Input: part model. Units: mm. Frame: model coordinates. A direction names the side the tool comes from. Round coordinates to 2 decimals unless told otherwise and drop trailing zeros. Loops run counter-clockwise (first coordinate to the right, second up) from the corner with the lowest first, then second, coordinate; pieces in that order, holes last. Notation, with made-up numbers: (23, 51) -> (42, 51) arc R7 cw to (42, 55) -> close; hole circle Ø7 at (39, 34.5). An arc over 180 degrees is marked (long way). Answer as a JSON object with one key per item and string values. Group by question number.
Item 1: Set-up query: faces 5 (the flat face through (155, 18, 3.175)), 6 (the flat face through (88, 0, 3)). Return all of +Z, -Z, +X, -X, +Y, -Y with unobstructed straight access to the full face (end or side cutting, diameter ignored); none if empty.
Item 2: Material intervals for line 1 (Y direction, x = 20, z = 4.65); line 2 (Z direction, x = 114.5, y = 15.25) (3 decimals), sorted ascending. Write a range as [from, to].
Item 3: Draft query along X for faces 1 (the flat face through (0, 13, 3)), 2 (the flat face through (115, 7, 3.175)), 3 (the flat face through (88, 13, 5.715)), 4 (the flat face through (76, 18, 3.175)). Return one class per face: released by +X, released by -X, zero draft, split by the parting line, or undercut.
Item 4: Section query B-B on z = 4.75. Count the separate pieces of the cut face and the enclosed holes in it, and give its area (3 significant figures).
Item 5: Pin query (flat end, axial travel): pin 1 (6 mm diameter, centred on x = 107, y = 6, fed in from -Z); pin 2 (3 mm diameter, centred on x = 62, y = 18, fed in from +Z) (3 decimals). Return the tip coordinate at first contact, or that it passes through.
Item 6: Section query A-A on x = 156. Return loops of the section in (y, z) (3 decimals).
from build123d import *

# Parameters (mm, degrees)
F0_W     = 177.8
F0_H     = 25.4
F1_DEPTH = 3.175
F2_W     = 177.8
F2_H     = 25.4
F2_W_2   = 6.489529
F2_H_2   = 6.479562
F3_DEPTH = 2.54


with BuildPart() as f1:
    # F0 (on Top) → F1 (new body)
    with BuildSketch(Plane.XY):
        with Locations((88.9, 12.7)):
            Rectangle(F0_W, F0_H)
    extrude(amount=F1_DEPTH)

    # F2 (on face) → F3 (join)
    with BuildSketch(Plane.XY.offset(3.175)):
        with Locations((88.9, 12.7)):
            Rectangle(F2_W, F2_H)
        with Locations((9.734293, 7.034986)):
            Rectangle(F2_W_2, F2_H_2, mode=Mode.SUBTRACT)
        with Locations((22.942293, 7.034986)):
            Rectangle(F2_W_2, F2_H_2, mode=Mode.SUBTRACT)
        with Locations((36.150294, 7.034986)):
            Rectangle(F2_W_2, F2_H_2, mode=Mode.SUBTRACT)
        with Locations((49.358294, 7.034986)):
            Rectangle(F2_W_2, F2_H_2, mode=Mode.SUBTRACT)
        with Locations((62.566294, 7.034986)):
            Rectangle(F2_W_2, F2_H_2, mode=Mode.SUBTRACT)
        with Locations((75.774293, 7.034986)):
            Rectangle(F2_W_2, F2_H_2, mode=Mode.SUBTRACT)
        with Locations((88.982293, 7.034986)):
            Rectangle(F2_W_2, F2_H_2, mode=Mode.SUBTRACT)
        with Locations((102.190293, 7.034986)):
            Rectangle(F2_W_2, F2_H_2, mode=Mode.SUBTRACT)
        with Locations((115.398293, 7.034986)):
            Rectangle(F2_W_2, F2_H_2, mode=Mode.SUBTRACT)
        with Locations((128.606293, 7.034986)):
            Rectangle(F2_W_2, F2_H_2, mode=Mode.SUBTRACT)
        with Locations((141.814293, 7.034986)):
            Rectangle(F2_W_2, F2_H_2, mode=Mode.SUBTRACT)
        with Locations((155.022293, 7.034986)):
            Rectangle(F2_W_2, F2_H_2, mode=Mode.SUBTRACT)
        with Locations((168.230293, 7.034986)):
            Rectangle(F2_W_2, F2_H_2, mode=Mode.SUBTRACT)
        with Locations((9.734293, 18.350219)):
            Rectangle(F2_W_2, F2_H_2, mode=Mode.SUBTRACT)
        with Locations((22.942293, 18.350219)):
            Rectangle(F2_W_2, F2_H_2, mode=Mode.SUBTRACT)
        with Locations((36.150294, 18.350219)):
            Rectangle(F2_W_2, F2_H_2, mode=Mode.SUBTRACT)
        with Locations((49.358294, 18.350219)):
            Rectangle(F2_W_2, F2_H_2, mode=Mode.SUBTRACT)
        with Locations((62.566294, 18.350219)):
            Rectangle(F2_W_2, F2_H_2, mode=Mode.SUBTRACT)
        with Locations((75.774293, 18.350219)):
            Rectangle(F2_W_2, F2_H_2, mode=Mode.SUBTRACT)
        with Locations((88.982293, 18.350219)):
            Rectangle(F2_W_2, F2_H_2, mode=Mode.SUBTRACT)
        with Locations((102.190293, 18.350219)):
            Rectangle(F2_W_2, F2_H_2, mode=Mode.SUBTRACT)
        with Locations((115.398293, 18.350219)):
            Rectangle(F2_W_2, F2_H_2, mode=Mode.SUBTRACT)
        with Locations((128.606293, 18.350219)):
            Rectangle(F2_W_2, F2_H_2, mode=Mode.SUBTRACT)
        with Locations((141.814293, 18.350219)):
            Rectangle(F2_W_2, F2_H_2, mode=Mode.SUBTRACT)
        with Locations((155.022293, 18.350219)):
            Rectangle(F2_W_2, F2_H_2, mode=Mode.SUBTRACT)
        with Locations((168.230293, 18.350219)):
            Rectangle(F2_W_2, F2_H_2, mode=Mode.SUBTRACT)
    extrude(amount=F3_DEPTH)


solid = f1.part
Solved:
{
 "1": {"face 5": "+Z", "face 6": "+Z, -Z, +X, -X, -Y"},
 "2": {"line 1": "[0, 3.8], [10.27, 15.11], [21.59, 25.4]", "line 2": "[0, 3.175]"},
 "3": {"face 1": "released by -X", "face 2": "undercut", "face 3": "zero draft", "face 4": "undercut"},
 "4": {"separate pieces": "1", "enclosed holes": "26", "area": "3,420 mm²"},
 "5": {"pin 1": "z = 0", "pin 2": "z = 3.175"},
 "6": {"outline": "(0, 0) -> (25.4, 0) -> (25.4, 5.715) -> (21.59, 5.715) -> (21.59, 3.175) -> (15.11, 3.175) -> (15.11, 5.715) -> (10.275, 5.715) -> (10.275, 3.175) -> (3.795, 3.175) -> (3.795, 5.715) -> (0, 5.715) -> close"}
}
